The listing builds one solid part. Answer for the finished solid, in the listing's coordinates (mm). A direction names the side the tool comes from. Give positions to 0.01 mm unless a question says otherwise; leave off trailing zeros. Order: outer loops, then holes, each group sorted by start corner. A loop starts at its lowest first (then second) coordinate and runs counter-clockwise, first axis right, second up. Notation, with made-up numbers: M 10.25,21.5 L 39.25,21.5 A7 ccw 39.25,30.5 Z; hole C -6,30 d10. An arc over 180 degrees is marked long. Answer as a JSON object with one key per item and string values. Group by question number.
```python
from build123d import *

# Parameters (mm, degrees)
SKETCH_1_R          = 15
EXTRUDE_1_DEPTH     = 20
SKETCH_2_R          = 45
EXTRUDE_2_DEPTH     = 20
SKETCH_3_R          = 7.65
CUT_EXTRUDE_1_DEPTH = 10


with BuildPart() as part:
    # 草图1 → 凸台-拉伸1 (new body, symmetric)
    with BuildSketch(Plane(origin=(0, 0, 0), x_dir=(1, 0, 0), z_dir=(0, 1, 0))):
        with BuildLine():
            Line((-30, 0), (-30, 50))
            ThreePointArc((-30, 50), (0, 80), (30, 50))
            Line((30, 50), (30, 0))
            Line((30, 0), (-30, 0))
        make_face()
        with Locations((0, 50)):
            Circle(SKETCH_1_R, mode=Mode.SUBTRACT)
    extrude(amount=EXTRUDE_1_DEPTH, both=True)

    # 草图2 → 凸台-拉伸2 (add)
    with BuildSketch(Plane.XY):
        Circle(SKETCH_2_R)
    extrude(amount=EXTRUDE_2_DEPTH)

    # 草图3 → 切除-拉伸1 (cut)
    with BuildSketch(Plane.XY.offset(20)):
        Circle(SKETCH_3_R)
    extrude(amount=-CUT_EXTRUDE_1_DEPTH, mode=Mode.SUBTRACT)


solid = part.part
```
Item 1: Section D-D (z = -14) is taken. Determine the outline of the cut face in (x, y).
Item 2: A tool of negligible diameter and unlimited length cuts with its end or side. For faces 4 (the flat face through (-30, 0, -25)), 5 (the flat face through (0, -20, -32)), 6 (the flat face through (0, 20, -32)), 7 (the flat face through (0, 0, 10)), 8 (the cylindrical face through (20.765, -39.923, 9.86)), from which of +Z, -Z, +X, -X, +Y, -Y can it reach the whole face along a straight path? Write none if from no direction.
Item 3: Consider probe 1 along X at (y, z) = (11, -50); probe 2 along Z at (x, y) = (0, 7); probe 3 along Y at (x, z) = (0, 16.25). Determine where each line is inside the solid, lowest interval first. Write a range as from..to.
Item 4: Section A-A (x = 0) is taken. Determine the outline of the cut face in (y, z).
Item 5: Section C-C (z = -47) is taken. Determine the outline of the cut face in (x, y), and give its area (3 significant figures).
Item 6: Flat-ended cylindrical pins translate along their axes: P1, Ø17.5, axis at x = 0, y = 0, coming from the -Z side; P2, Ø3, axis at y = -10.5, z = -6.5, coming from the +X side; P3, Ø6, axis at x = -35, y = -17.5, coming from the -Z side. Find the tip coordinate at first contact, or state that the pin passes through.
Item 7: Section B-B (y = 0) is taken. Determine the outline of the cut face in (x, z).
Item 8: Determine the mould class of faces 1 (the flat face through (-1, -9, 20)), 2 (the flat face through (30, 0, -25)), 3 (the cylindrical face through (-1.953, -0.28, -64.872)) for opening direction X: released by +X, released by -X, zero draft, split by the parting line, or undercut.
Values found:
{
 "1": {"outline": "M -30,-20 L 30,-20 L 30,20 L -30,20 Z"},
 "2": {"face 4": "-Z, -X, +Y, -Y", "face 5": "-Z, +X, -X, -Y", "face 6": "-Z, +X, -X, +Y", "face 7": "+Z", "face 8": "+Z, -Z"},
 "3": {"probe 1": "x = -30..-15, 15..30", "probe 2": "z = -80..-65, -35..10", "probe 3": "y = -45..-7.65, 7.65..45"},
 "4": {"outline": "M -45,0 L -20,0 L -20,-35 L 20,-35 L 20,0 L 45,0 L 45,20 L 7.65,20 L 7.65,10 L -7.65,10 L -7.65,20 L -45,20 Z; M -20,-80 L 20,-80 L 20,-65 L -20,-65 Z"},
 "5": {"outline": "M -30,-20 L -14.7,-20 L -14.7,20 L -30,20 Z; M 14.7,-20 L 30,-20 L 30,20 L 14.7,20 Z", "area": "1,220 mm^2"},
 "6": {"P1": "stops at z = -80", "P2": "stops at x = 30", "P3": "stops at z = 0"},
 "7": {"outline": "M -45,0 L -30,0 L -30,-50 A30 ccw 30,-50 L 30,0 L 45,0 L 45,20 L 7.65,20 L 7.65,10 L -7.65,10 L -7.65,20 L -45,20 Z; hole C 0,-50 d30"},
 "8": {"face 1": "zero draft", "face 2": "released by +X", "face 3": "undercut"}
}
